Part print with two shaded views. Sizes in mm from the minimum x, y, z corner. A direction names the side the tool comes from. Round coordinates to 2 decimals unless told otherwise and drop trailing zeros. Write each loop counter-clockwise with the first axis right and the second up, starting at its lowest first coordinate (ties: lowest second). Pieces come first, ordered by that corner, then holes. Notation, with made-up numbers: (7, 5) - (53, 5) arc R20 ccw to (53, 31) - close; hole circle Ø11 at (58, 66.25). An arc over 180 degrees is marked (long way). Answer as a JSON object with one key per item and string values. Group by question number.
Item 1: Probe line 1 (X direction, y = 7.75, z = 23.5); line 2 (Z direction, x = 37, y = 7.5); line 3 (X direction, y = 1, z = 4.5). List the from-to ranges inside material, lowest first. Write a range as from..to.
Item 2: Slice it at B-B, the plane y = 6. List the corners of the cut face in (x, z), then the cut area to 3 significant figures.
Item 3: Slice it at A-A, the plane z = 34. List the corners of the cut face in (x, y).
Item 4: Which spindle directions (+Z, -Z, +X, -X, +Y, -Y) get a long thin tool onto all of the face, cutting with end or side? Do the marked faces 1, 2 and 3. Say none if no direction does.
Item 5: Flat gauge pins, fed straight in: pin 1 (1.8 mm diameter, centred on y = 5.5, z = 24, fed in from -X); pin 2 (1.5 mm diameter, centred on y = 7, z = 20, fed in from +X); pin 3 (2.5 mm diameter, centred on x = 127, z = 17.5, fed in from +Y). Where does each tip first touch, or does it go through?
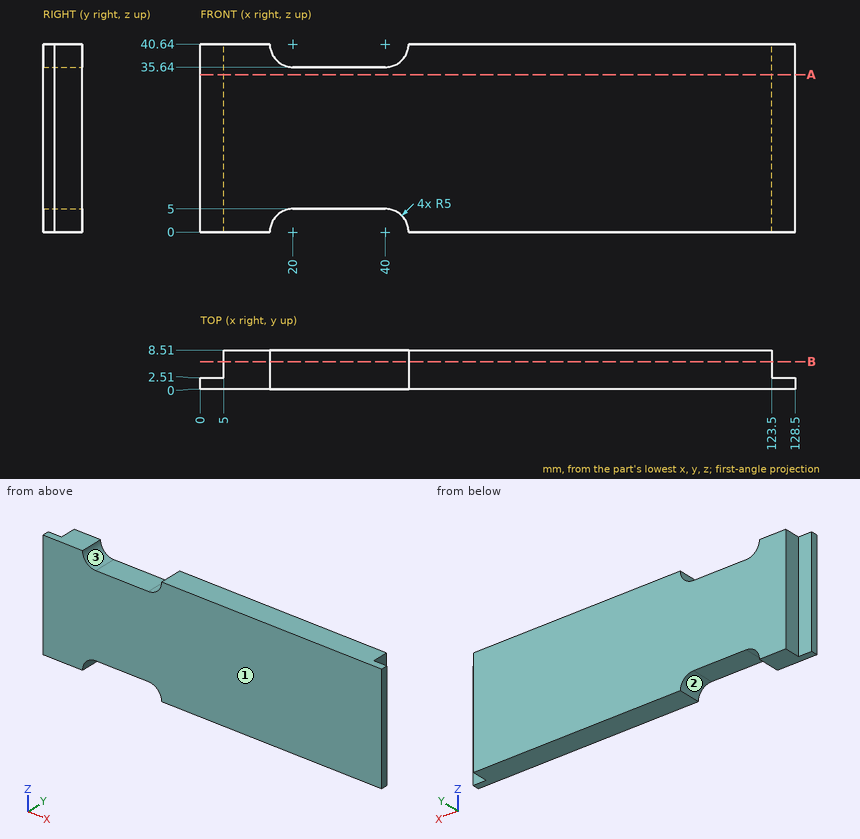
Geometry says:
{
 "1": {"line 1": "x = 5..123.5", "line 2": "z = 5..35.64", "line 3": "x = 0..17.82, 42.18..128.5"},
 "2": {"outline": "(5, 0) - (15, 0) arc R5 cw to (20, 5) - (40, 5) arc R5 cw to (45, 0) - (123.5, 0) - (123.5, 40.64) - (45, 40.64) arc R5 cw to (40, 35.64) - (20, 35.64) arc R5 cw to (15, 40.64) - (5, 40.64) - close", "area": "4,540 mm^2"},
 "3": {"outline": "(0, 0) - (128.5, 0) - (128.5, 2.51) - (123.5, 2.51) - (123.5, 8.51) - (5, 8.51) - (5, 2.51) - (0, 2.51) - close"},
 "4": {"face 1": "+Z, -Z, +X, -X, -Y", "face 2": "-Z, +Y, -Y", "face 3": "+Z, +Y, -Y"},
 "5": {"pin 1": "stops at x = 5", "pin 2": "stops at x = 123.5", "pin 3": "stops at y = 2.51"}
}
